```python
from build123d import *

# Parameters (mm, degrees)
F1_DEPTH    = 38.1
F2_R        = 10.16
F3_R        = 10.16
F5_DEPTH    = 6.35
F6_W        = 3.8326773793
F6_H        = 31.7183228926
F6_W_2      = 4.029225558
F6_W_3      = 4.3240477098
F6_W_4      = 4.6188691631
F6_W_5      = 4.6188682318
F6_W_6      = 4.4223219156
F7_DEPTH    = 2.794
F8_T1_DEPTH = 43.1483228926


# Not quite as in the source:
# - a fillet or chamfer that OpenCascade refuses, or shapes differently, is made with other operations: its cross-section is extruded or revolved along the edge and cut away or added


with BuildPart() as f1:
    # F0 (on Top) → F1 (new body)
    with BuildSketch(Plane.XY):
        Polygon((-33.02, -26.0191614463), (32.2342477739, -26.0191614463), (52.0383228926, -10.6488130987), (52.0383228926, 10.6521614463), (32.2342477739, 26.0191614463), (-33.02, 26.0191614463), (-52.0383228926, 10.6521614463), (-52.0383228926, -10.6488130987), align=None)
    extrude(amount=F1_DEPTH)

    # F2
    f2_edges = [f1.edges().sort_by_distance(p)[0] for p in [
        (-0.392876, -26.019161, 38.1),
        (-42.529161, -18.333987, 38.1),
        (-52.038323, 0.001674, 38.1),
        (-42.529161, 18.335661, 38.1),
        (-0.392876, 26.019161, 38.1),
        (42.136285, 18.335661, 38.1),
        (52.038323, 0.001674, 38.1),
        (42.136285, -18.333987, 38.1),
    ]]
    fillet(f2_edges, radius=F2_R)

    # F3
    f3_edges = [f1.edges().sort_by_distance(p)[0] for p in [
        (-0.392876, -26.019161, 0),
        (-42.529161, -18.333987, 0),
        (-52.038323, 0.001674, 0),
        (-42.529161, 18.335661, 0),
        (-0.392876, 26.019161, 0),
        (42.136285, 18.335661, 0),
        (52.038323, 0.001674, 0),
        (42.136285, -18.333987, 0),
    ]]
    fillet(f3_edges, radius=F3_R)

    # F4 (on face) → F5 (join)
    with BuildSketch(Plane.XY.offset(38.1)):
        Polygon((-29.4282840059, 15.8591614463), (-41.8783228926, 5.7994023049), (-41.8783228926, -5.7967184312), (-29.4276753196, -15.8591614463), (28.7541399654, -15.8591614463), (41.8783228926, -5.6732142531), (41.8783228926, 5.6758979589), (28.7547389102, 15.8591614463), align=None)
    extrude(amount=F5_DEPTH)

    # F6 (on face) → F7 (join)
    with BuildSketch(Plane.XY.offset(44.45)):
        with Locations((-22.4555665627, 0)):
            Rectangle(F6_W, F6_H)
        with Locations((-12.9230059683, 0)):
            Rectangle(F6_W_2, F6_H)
        with Locations((-3.4395834082, 0)):
            Rectangle(F6_W_3, F6_H)
        with Locations((5.8472915553, 0)):
            Rectangle(F6_W_4, F6_H)
        with Locations((15.0850303471, 0)):
            Rectangle(F6_W_5, F6_H)
        with Locations((22.6521138102, 0)):
            Rectangle(F6_W_6, F6_H)
    extrude(amount=F7_DEPTH)

    # F8: fillet of radius 2.286 on 12 edges, made by hand

    # F8_s2 → F8_t1 (cut)
    with BuildSketch(Plane.XZ.offset(-21.5741614463)):
        with BuildLine():
            ThreePointArc((-20.5392278731, 44.958), (-21.2087817713, 46.5744461018), (-22.8252278731, 47.244))
            Line((-22.8252278731, 47.244), (-20.5392278731, 47.244))
            Line((-20.5392278731, 47.244), (-20.5392278731, 44.958))
        make_face()
        with BuildLine():
            ThreePointArc((-10.9083931893, 44.958), (-11.5779470875, 46.5744461018), (-13.1943931893, 47.244))
            Line((-13.1943931893, 47.244), (-10.9083931893, 47.244))
            Line((-10.9083931893, 47.244), (-10.9083931893, 44.958))
        make_face()
        with BuildLine():
            ThreePointArc((-1.2775595533, 44.958), (-1.9471134515, 46.5744461018), (-3.5635595533, 47.244))
            Line((-3.5635595533, 47.244), (-1.2775595533, 47.244))
            Line((-1.2775595533, 47.244), (-1.2775595533, 44.958))
        make_face()
        with BuildLine():
            ThreePointArc((8.1567261368, 44.958), (7.4871722386, 46.5744461018), (5.8707261368, 47.244))
            Line((5.8707261368, 47.244), (8.1567261368, 47.244))
            Line((8.1567261368, 47.244), (8.1567261368, 44.958))
        make_face()
        with BuildLine():
            ThreePointArc((17.394464463, 44.958), (16.7249105648, 46.5744461018), (15.108464463, 47.244))
            Line((15.108464463, 47.244), (17.394464463, 47.244))
            Line((17.394464463, 47.244), (17.394464463, 44.958))
        make_face()
        with BuildLine():
            ThreePointArc((24.863274768, 44.958), (24.1937208698, 46.5744461018), (22.577274768, 47.244))
            Line((22.577274768, 47.244), (24.863274768, 47.244))
            Line((24.863274768, 47.244), (24.863274768, 44.958))
        make_face()
        with BuildLine():
            ThreePointArc((20.4409528524, 44.958), (21.1105067506, 46.5744461018), (22.7269528524, 47.244))
            Line((22.7269528524, 47.244), (20.4409528524, 47.244))
            Line((20.4409528524, 47.244), (20.4409528524, 44.958))
        make_face()
        with BuildLine():
            ThreePointArc((12.7755962312, 44.958), (13.4451501294, 46.5744461018), (15.0615962312, 47.244))
            Line((15.0615962312, 47.244), (12.7755962312, 47.244))
            Line((12.7755962312, 47.244), (12.7755962312, 44.958))
        make_face()
        with BuildLine():
            ThreePointArc((3.5378569737, 44.958), (4.2074108719, 46.5744461018), (5.8238569737, 47.244))
            Line((5.8238569737, 47.244), (3.5378569737, 47.244))
            Line((3.5378569737, 47.244), (3.5378569737, 44.958))
        make_face()
        with BuildLine():
            ThreePointArc((-5.6016072631, 44.958), (-4.9320533649, 46.5744461018), (-3.3156072631, 47.244))
            Line((-3.3156072631, 47.244), (-5.6016072631, 47.244))
            Line((-5.6016072631, 47.244), (-5.6016072631, 44.958))
        make_face()
        with BuildLine():
            ThreePointArc((-14.9376187474, 44.958), (-14.2680648491, 46.5744461018), (-12.6516187474, 47.244))
            Line((-12.6516187474, 47.244), (-14.9376187474, 47.244))
            Line((-14.9376187474, 47.244), (-14.9376187474, 44.958))
        make_face()
        with BuildLine():
            ThreePointArc((-24.3719052523, 44.958), (-23.7023513541, 46.5744461018), (-22.0859052523, 47.244))
            Line((-22.0859052523, 47.244), (-24.3719052523, 47.244))
            Line((-24.3719052523, 47.244), (-24.3719052523, 44.958))
        make_face()
    extrude(amount=F8_T1_DEPTH, mode=Mode.SUBTRACT)


solid = f1.part
```
Here's how the part is built. I have some questions about the finished solid (model axes, mm). A direction names the side the tool comes from. Round coordinates to 2 decimals unless told otherwise and drop trailing zeros. Order: outer loops, then holes, each group sorted by start corner. A loop starts at its lowest first (then second) coordinate and runs counter-clockwise, first axis right, second up. Notation, with made-up numbers: M -29.5,51.25 L -11.5,51.25 A15 cw -11.5,65.25 Z; hole C 36,56.25 d9. An arc over 180 degrees is marked long. One line per question, with ' | ' between items.
1) I need wall thicknesses on line 1 along Z through (x, y) = (23, 4); line 2 along Z through (x, y) = (17.5, -4); line 3 along Y through (x, z) = (-18.5, 44). Which ranges of each line are inside material? Lowest first, please.
Working result:
line 1: 0 to 47.2 | line 2: 0 to 44.45 | line 3: -15.86 to 15.86
2) If we mould it in two halves opening along X, with no side actions, what happens to faces 5 (the face through (42, -18.44, 18.93)), 6 (the face through (19, 0, 44.45)), 7 (the face through (7.5, 0.22, 46.56)), 8 (the face through (-41.878, 0, 41))? For each: +X half, -X half, draft (parallel to the pull), parting line (faces both ways), or undercut.
Working result:
face 5: +X half | face 6: undercut | face 7: undercut | face 8: -X half
3) I want a section at B-B, the plane z = 42. Write out the boundary of the cut face in (x, y), then the cut area to 3 significant figures.
Working result:
outline: M -41.88,-5.8 L -29.43,-15.86 L 28.75,-15.86 L 41.88,-5.67 L 41.88,5.68 L 28.75,15.86 L -29.43,15.86 L -41.88,5.8 Z | area: 2,400 mm²
4) For faces 1 (the face through (-14.377, 0.222, 46.458)), 2 (the face through (-35.566, 10.9, 41.231)), 3 (the face through (31, 0, 44.45)), 4 (the face through (-31, 0, 44.45)), which set-ups out of +Z, -Z, +X, -X, +Y, -Y let a thin tool reach every point of the face, with its end or its side?
Working result:
face 1: +Z, +Y, -Y | face 2: +Z, -X, +Y | face 3: +Z, +X, +Y, -Y | face 4: +Z, -X, +Y, -Y
5) I want a section at A-A, the plane z = 11.5. Write out the boundary of the cut face in (x, y).
Working result:
outline: M -52.04,-10.65 L -33.02,-26.02 L 32.23,-26.02 L 52.04,-10.65 L 52.04,10.65 L 32.23,26.02 L -33.02,26.02 L -52.04,10.65 Z
6) For pin 1 Ø0.6 at (y, z) = (5.5, 44.5) entering from -X; pin 2 Ø10 at (y, z) = (-17.5, 23) entering from -X; pin 3 Ø4 at (x, z) = (-39.5, 7.5) entering from -Y, each with a flat end and sliding along its axis, tell me the tip position at first contact or that it passes through.
Working result:
pin 1: x = -41.88 | pin 2: x = -49.75 | pin 3: y = -22.05
